```python
from build123d import *

# Parameters (mm, degrees)
SKETCH2_R           = 20
SKETCH2_W           = 40.133980871
SKETCH2_H           = 98.510680321
BOSS_EXTRUDE1_DEPTH = 10
SKETCH3_W           = 26.229690347
SKETCH3_H           = 62.525074854
BOSS_EXTRUDE2_DEPTH = 1
SKETCH4_R           = 5
BOSS_EXTRUDE3_DEPTH = 15
SKETCH5_W           = 32.37828677
SKETCH5_H           = 23.159469009
BOSS_EXTRUDE4_DEPTH = 20
SKETCH6_R           = 9
SKETCH6_R_2         = 8
BOSS_EXTRUDE5_DEPTH = 4
SKETCH7_R           = 1.505673325
BOSS_EXTRUDE6_DEPTH = 13


with BuildPart() as part:
    # Sketch1 → Revolve2 (revolve)
    with BuildSketch(Plane(origin=(0, 0, 0), x_dir=(0, 0, -1), z_dir=(1, 0, 0)), mode=Mode.PRIVATE) as revolve2_sk:
        Polygon((-124.727272727, 4.929753727), (-120, 4.929753727), (-120, 0.318181818), (-52.5, 0.318181818), (-52.5, 4.929753727), (-50.5, 4.929753727), (-50.5, 12.318181818), (-50.5, 22.651670955), (-3.5, 22.651670955), (-3.5, 28.996436074), (-50.5, 28.996436074), (-55.732846455, 28.996436074), (-55.732846455, 12.318181818), (-124.727272727, 12.318181818), align=None)
    revolve(revolve2_sk.sketch.rotate(Axis((0, -1000, 0), (0, 1, 0)), 180), axis=Axis((0, -1000, 0), (0, 1, 0)))

    # Sketch2 → Boss-Extrude1 (add)
    with BuildSketch(Plane(origin=(0, 12.318181818, 0), x_dir=(1, 0, 0), z_dir=(0, 1, 0))):
        with Locations(Location((0, 94.391996497, 0), (0, 0, 90))):
            Circle(SKETCH2_R)
        with Locations((86.897306122, -2.763043919)):
            Rectangle(SKETCH2_W, SKETCH2_H)
    extrude(amount=BOSS_EXTRUDE1_DEPTH)

    # Sketch3 → Boss-Extrude2 (add)
    with BuildSketch(Plane(origin=(0, 22.318181818, 0), x_dir=(1, 0, 0), z_dir=(0, 1, 0))):
        with Locations((83.554770675, -17.111809319)):
            Rectangle(SKETCH3_W, SKETCH3_H)
    extrude(amount=BOSS_EXTRUDE2_DEPTH)

    # Sketch4 → Boss-Extrude3 (add)
    with BuildSketch(Plane(origin=(0, 22.318181818, 0), x_dir=(1, 0, 0), z_dir=(0, 1, 0))):
        with Locations(Location((0, 107.827495102, 0), (0, 0, 270))):
            Circle(SKETCH4_R)
    extrude(amount=BOSS_EXTRUDE3_DEPTH)

    # Sketch5 → Boss-Extrude4 (add)
    with BuildSketch(Plane(origin=(0, 22.318181818, 0), x_dir=(1, 0, 0), z_dir=(0, 1, 0))):
        with Locations((87.532995765, 31.614032761)):
            Rectangle(SKETCH5_W, SKETCH5_H)
    extrude(amount=BOSS_EXTRUDE4_DEPTH)

    # Sketch6 → Boss-Extrude5 (add)
    with BuildSketch(Plane(origin=(103.72213915, 0, 0), x_dir=(0, 0, -1), z_dir=(1, 0, 0))):
        with Locations(Location((31.614032762, 32.318181818, 0), (0, 0, 180))):
            Circle(SKETCH6_R)
        with Locations((31.614032762, 32.318181818)):
            Circle(SKETCH6_R_2, mode=Mode.SUBTRACT)
    extrude(amount=BOSS_EXTRUDE5_DEPTH)

    # Sketch7 → Boss-Extrude6 (add)
    with BuildSketch(Plane(origin=(103.72213915, 0, 0), x_dir=(0, 0, -1), z_dir=(1, 0, 0))):
        with Locations(Location((34.758166352, 35.526981806, 0), (0, 0, 180))):
            Circle(SKETCH7_R)
        with Locations(Location((28.469899171, 35.526981806, 0), (0, 0, 180))):
            Circle(SKETCH7_R)
        with Locations(Location((34.758166352, 29.10938183, 0), (0, 0, 180))):
            Circle(SKETCH7_R)
        with Locations(Location((28.469899171, 29.10938183, 0), (0, 0, 180))):
            Circle(SKETCH7_R)
    extrude(amount=BOSS_EXTRUDE6_DEPTH)


solid = part.part
```
Read the model definition and answer for the solid it produces. Units are mm, in the model's axes. A direction names the side the tool comes from. Give positions to 0.01 mm unless a question says otherwise; leave off trailing zeros. Loops run counter-clockwise (first coordinate to the right, second up) from the corner with the lowest first, then second, coordinate; pieces in that order, holes last.
Item 1: Find the intervals of material crossed by line 1 along X through (y, z) = (18.75, 0); line 2 along Y through (x, z) = (109, -35); line 3 along X through (y, z) = (10.5, 0), in increasing order.
Item 2: For faces 1 (the cylindrical face through (49.3, 13.91, 10.95)), 2 (the flat face through (66.83, 17, 3)), 3 (the cylindrical face through (49.445, 20.541, -25.717)), determine the directions among +Z, -Z, +X, -X, +Y, -Y from which every point of the face is accessible in a straight line to the end or side of a thin tool.
Item 3: The mould has two halves that part along X. Classify faces 4 (the cylindrical face through (105.694, 37.725, -25.718)), 5 (the flat face through (-43, 4.93, 27)), 6 (the cylindrical face through (-101.184, 2.592, -64.511)), 7 (the flat face through (11, 22.652, 1)): released by +X, released by -X, zero draft, split by the parting line, or undercut.
Item 4: Each of these flat-tipped pins is pushed along its axis until it touches: pin 1 Ø0.5 at (y, z) = (22.5, 14.5) entering from -X; pin 2 Ø6 at (y, z) = (28.5, -31.5) entering from +X; pin 3 Ø0.8 at (y, z) = (23, 9) entering from +X. Where does it stop, or does it pass through?
Item 5: The part is cut by section A-A (y = 19). Write down the section's boundary in (x, z), and give its area (3 significant figures).
Item 6: The part is cut by section D-D (z = -61). Write down the section's boundary in (x, y), and give its area (3 significant figures).
Taken from the geometry:
1. line 1: x = -55.73 to -50.5, 50.5 to 55.73, 66.83 to 106.96
1. line 2: y = 0.32 to 12.32, 27.62 to 30.6, 34.04 to 37.01
1. line 3: x = -124.73 to -50.5, 50.5 to 124.73
2. face 1: -Y
2. face 2: +Z, -Z, +Y
2. face 3: +Y
3. face 4: zero draft
3. face 5: undercut
3. face 6: split by the parting line
3. face 7: undercut
4. pin 1: stops at x = -53.88
4. pin 2: stops at x = 116.72
4. pin 3: stops at x = 96.67
5. outline: circle Ø111.47 at (0, 0); circle Ø40 at (0, -94.39); (66.83, -46.49) - (106.96, -46.49) - (106.96, 52.02) - (66.83, 52.02) - close; hole circle Ø101 at (0, 0)
5. area: 6,960 mm2
6. outline: (-108.79, 4.93) - (-103.34, 4.93) - (-103.34, 0.32) - (103.34, 0.32) - (103.34, 4.93) - (108.79, 4.93) - (108.79, 12.32) - (-108.79, 12.32) - close
6. area: 2,560 mm2
